The model under review builds one solid part; all positions refer to its coordinate system, in mm. Face numbers are marked on the shaded views. A direction names the side the tool comes from. Coordinates: 2 decimals unless noted, no trailing zeros. Write each loop counter-clockwise with the first axis right and the second up, starting at its lowest first coordinate (ties: lowest second). Pieces come first, ordered by that corner, then holes. Notation, with made-up numbers: (-32, 23) - (-20, 23) arc R18 ccw to (-20, 42) - close; hole circle Ø5 at (-33, -7.75). An arc over 180 degrees is marked (long way). Answer as CSV lines item,"result". Start each with the question number.
```python
from build123d import *

# Parameters (mm, degrees)
EXTRUDE_1_DEPTH = 2
SKETCH_2_R      = 1.5
EXTRUDE_2_DEPTH = 8
CHAMFER_1_SIZE  = 0.5


with BuildPart() as part:
    # Эскиз1 → Вытянуть1 (new body)
    with BuildSketch(Plane.XY):
        Polygon((0, 3.175426481), (-2.75, 1.58771324), (-2.75, -1.58771324), (0, -3.175426481), (2.75, -1.58771324), (2.75, 1.58771324), align=None)
    extrude(amount=EXTRUDE_1_DEPTH)

    # Эскиз2 → Вытянуть2 (add)
    with BuildSketch(Plane(origin=(0, 0, 0), x_dir=(-1, 0, 0), z_dir=(0, 0, -1))):
        with Locations(Location((0, 0, 0), (0, 0, 180))):
            Circle(SKETCH_2_R)
    extrude(amount=EXTRUDE_2_DEPTH)

    # Эскиз15 → Вырез-Повернуть1 (revolve, cut)
    with BuildSketch(Plane(origin=(0, 0, 0), x_dir=(0, 0, -1), z_dir=(1, 0, 0))):
        Polygon((-2, 3.175426481), (-2, 2.787926481), (-1.6125, 3.175426481), align=None)
    revolve(axis=Axis((0, 0, 4.465296569), (0, 0, -1)), mode=Mode.SUBTRACT)

    # Фаска1
    chamfer_1_edges = [part.edges().sort_by_distance(p)[0] for p in [
        (-1.5, 0, -8),
    ]]
    chamfer(chamfer_1_edges, length=CHAMFER_1_SIZE)


solid = part.part
```
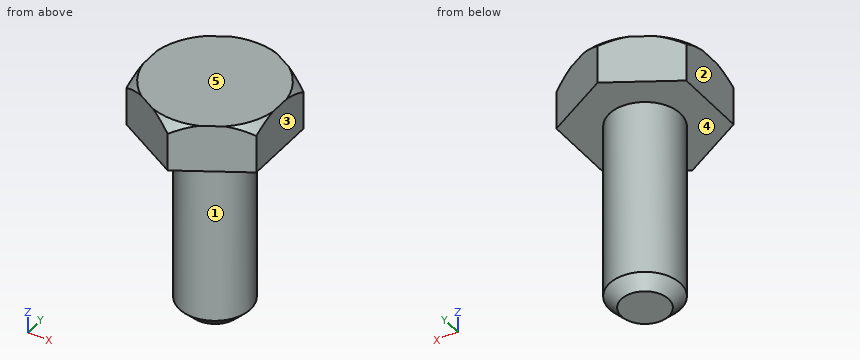
(1) Add section A-A on y = 0. Give the boundary of the cut face in (x, z), then the cut area to 4 significant figures.
(2) For the marked faces 1 and 2, list the 3-axis set-ups (+Z, -Z, +X, -X, +Y, -Y) from which the entire face can be reached by the end or side of a thin tool; tool diameter is ignored.
(3) Wall thickness on line 1 (Z direction, x = -1.5, y = 2); line 2 (Y direction, x = 0.05, z = -3); line 3 (Z direction, x = 0.25, y = 3): over which ranges is each line inside the solid? List them lowest first.
(4) For pin 1 (3 mm diameter, centred on x = 1, y = -2, fed in from -Z); pin 2 (2 mm diameter, centred on y = 1, z = -6.5, fed in from +X); pin 3 (3 mm diameter, centred on y = 1.5, z = -6, fed in from -X), all flat-tipped, find the tip position at first contact; note any pin that passes through.
(5) The part is to be moulded in two halves that separate along Z. For the marked faces 3, 4 and 5, say which applies: released by +Z, released by -Z, zero draft, split by the parting line, or undercut.
(6) Add section B-B on z = -5.75. Give the boundary of the cut face in (x, y), then the cut area to 3 significant figures.
Reported:
1,outline,"(-2.75, 0) - (-1.5, 0) - (-1.5, -7.5) - (-1, -8) - (1, -8) - (1.5, -7.5) - (1.5, 0) - (2.75, 0) - (2.75, 2) - (-2.75, 2) - close"
1,area,"34.75 mm²"
2,face 1,"-Z"
2,face 2,"+Z, -Z, -X, +Y, -Y"
3,line 1,"0 to 2"
3,line 2,"-1.5 to 1.5"
3,line 3,"0 to 1.78"
4,pin 1,"z = -8"
4,pin 2,"x = 1.5"
4,pin 3,"x = -1.5"
5,face 3,"zero draft"
5,face 4,"released by -Z"
5,face 5,"released by +Z"
6,outline,"circle Ø3 at (0, 0)"
6,area,"7.07 mm²"
